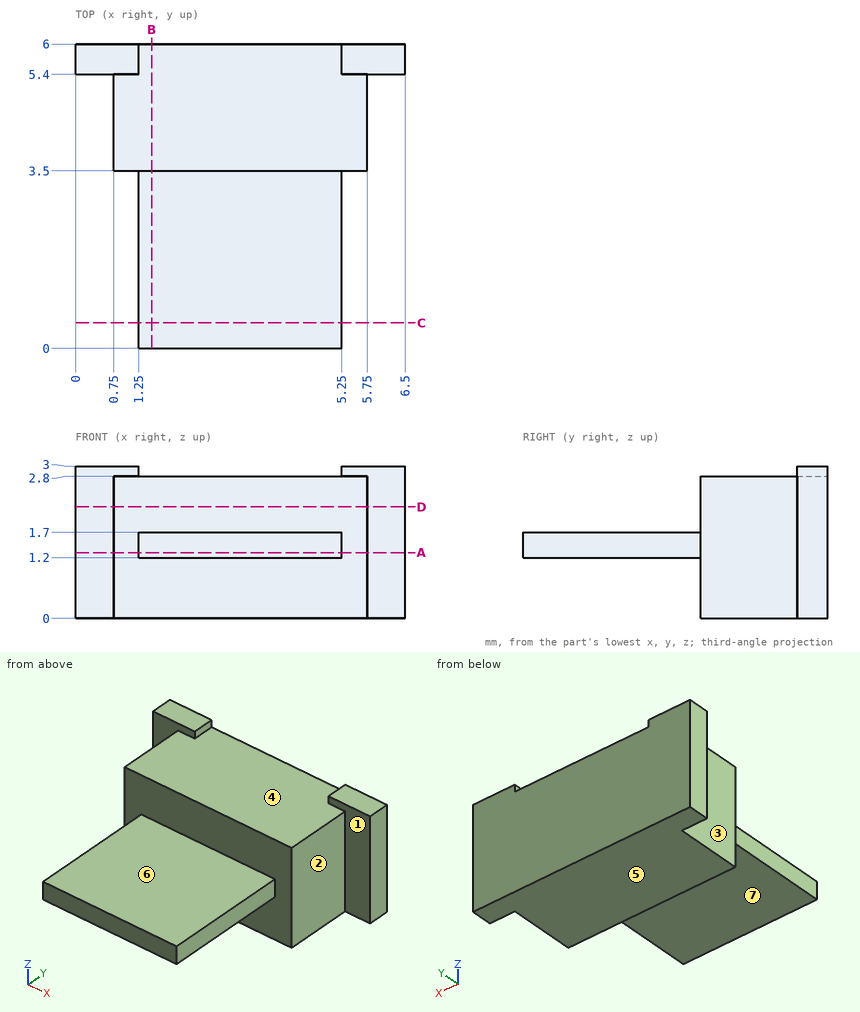
Check sheet for the drawn part. Datum: minimum x, y, z corner. Units: mm. A direction names the side the tool comes from. Coordinates: 2 decimals unless noted, no trailing zeros. Order: outer loops, then holes, each group sorted by start corner. A loop starts at its lowest first (then second) coordinate and runs counter-clockwise, first axis right, second up. Notation, with made-up numbers: (35.25, 37.25) -> (71.25, 37.25) arc R32 ccw to (71.25, 67.25) -> close; hole circle Ø6 at (-12, -11). An arc over 180 degrees is marked (long way). Use a Markdown table: item, result. Add a question column.
1. Mould release check, pull along X, two halves, no side actions. Record for the marked faces 1, 2, 3 and 4: pulls with the +X half, pulls with the -X half, needs draft (parallel to the pull), parting line crosses it, or undercut.
2. Cross-section at C-C (y = 0.5). Enter the section's corners in (x, z).
3. Cross-section at B-B (x = 1.5). Enter the section's corners in (y, z).
4. Material ranges on L1, parallel to Z at x = 4, y = 1.05; L2, parallel to X at y = 5.1, z = 1.9; L3, parallel to Z at x = 2.75, y = 4, recorded low to high.
5. Go/stop test with flat-tipped pins: pin 1 Ø1.4 at (x, z) = (6, 2) entering from -Y; pin 2 Ø1.5 at (y, z) = (4.5, 1.5) entering from +X; pin 3 Ø1.5 at (y, z) = (4, 2) entering from -X. Record where each tip stops, or that it passes through.
6. Cross-section at D-D (z = 2.2). Enter the section's corners in (x, y).
7. Cross-section at A-A (z = 1.3). Enter the section's corners in (x, y).
8. Set-up check for the marked faces 5, 6 and 7: record each of +Z, -Z, +X, -X, +Y, -Y from which the full face is reachable in a straight line by a thin tool's end or side.
Filled sheet:
| question | item | result |
|---|---|---|
| 1 | face 1 | needs draft |
| 1 | face 2 | pulls with the +X half |
| 1 | face 3 | pulls with the -X half |
| 1 | face 4 | undercut |
| 2 | outline | (1.25, 1.2) -> (5.25, 1.2) -> (5.25, 1.7) -> (1.25, 1.7) -> close |
| 3 | outline | (0, 1.2) -> (3.5, 1.2) -> (3.5, 0) -> (6, 0) -> (6, 2.8) -> (3.5, 2.8) -> (3.5, 1.7) -> (0, 1.7) -> close |
| 4 | L1 | 1.2 to 1.7 |
| 4 | L2 | 0.75 to 5.75 |
| 4 | L3 | 0 to 2.8 |
| 5 | pin 1 | y = 3.5 |
| 5 | pin 2 | x = 5.75 |
| 5 | pin 3 | x = 0.75 |
| 6 | outline | (0, 5.4) -> (0.75, 5.4) -> (0.75, 3.5) -> (5.75, 3.5) -> (5.75, 5.4) -> (6.5, 5.4) -> (6.5, 6) -> (0, 6) -> close |
| 7 | outline | (0, 5.4) -> (0.75, 5.4) -> (0.75, 3.5) -> (1.25, 3.5) -> (1.25, 0) -> (5.25, 0) -> (5.25, 3.5) -> (5.75, 3.5) -> (5.75, 5.4) -> (6.5, 5.4) -> (6.5, 6) -> (0, 6) -> close |
| 8 | face 5 | -Z, +X, -X, +Y, -Y |
| 8 | face 6 | +Z, +X, -X, -Y |
| 8 | face 7 | -Z, +X, -X, -Y |
